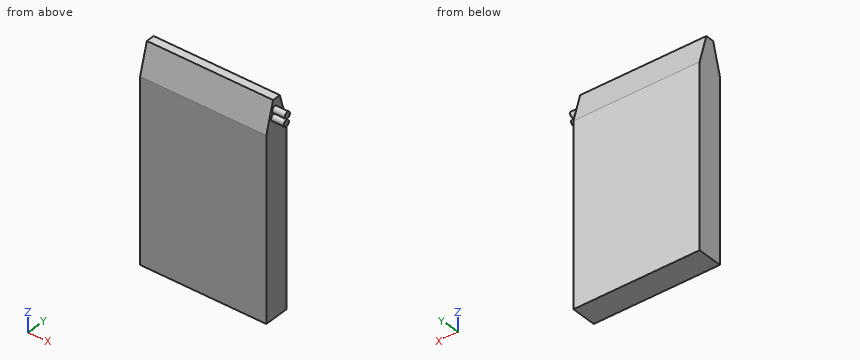
```python
from build123d import *

# Parameters (mm, degrees)
SKETCH1_W           = 30
SKETCH1_H           = 50
BOSS_EXTRUDE1_DEPTH = 6
CHAMFER1_SIZE       = 2
CHAMFER1_SIZE2      = 7
SKETCH2_R           = 0.75
BOSS_EXTRUDE2_DEPTH = 3


with BuildPart() as part:
    # Sketch1 → Boss-Extrude1 (new body)
    with BuildSketch(Plane(origin=(0, 0, 0), x_dir=(1, 0, 0), z_dir=(0, 1, 0))):
        Rectangle(SKETCH1_W, SKETCH1_H)
    extrude(amount=BOSS_EXTRUDE1_DEPTH)

    # Chamfer1
    chamfer1_edges = [part.edges().sort_by_distance(p)[0] for p in [
        (0, 0, 25),
        (0, 6, 25),
    ]]
    chamfer1_side = [part.faces().sort_by_distance(p)[0] for p in [
        (0, 3, 25),
    ]]
    chamfer(chamfer1_edges, length=CHAMFER1_SIZE, length2=CHAMFER1_SIZE2, reference=chamfer1_side[0])

    # Sketch2 → Boss-Extrude2 (add)
    with BuildSketch(Plane(origin=(15, 0, 0), x_dir=(0, 0, -1), z_dir=(1, 0, 0))):
        with Locations((-22.591828887, 2.491974932)):
            Circle(SKETCH2_R)
        with Locations((-20.930691136, 2.177979382)):
            Circle(SKETCH2_R)
    extrude(amount=BOSS_EXTRUDE2_DEPTH)


solid = part.part
```
For this review, take the finished solid that the model builds, in its own axes (mm). Coordinates: 2 decimals unless noted, no trailing zeros. Loops run counter-clockwise (first coordinate to the right, second up) from the corner with the lowest first, then second, coordinate; pieces in that order, holes last.
1. For line 1 (X direction, y = 4.5, z = 8); line 2 (Y direction, x = -6, z = 21.5), list the stretches that pass through material, from the lowest coordinate up.
2. Add section B-B, the plane z = 0. Give the boundary of the cut face in (x, y), then the cut area to 3 significant figures.
3. Add section C-C, the plane x = 16. Give the boundary of the cut face in (y, z), then the cut area to 3 significant figures.
4. Add section A-A, the plane x = -1. Give the boundary of the cut face in (y, z).
5. Add section D-D, the plane y = 4.75. Give the boundary of the cut face in (x, z) (3 decimals), then the cut area to 3 significant figures.
6. Insertion check: P1, Ø3, axis at y = 4.5, z = -5.5, coming from the +X side. The pin has a flat end and moves straight along its axis. Give the tip position at first contact, or say it passes through.
Result:
1. line 1: x = -15 to 15
1. line 2: y = 1 to 5
2. outline: (-15, 0) - (15, 0) - (15, 6) - (-15, 6) - close
2. area: 180 mm2
3. outline: circle Ø1.5 at (2.18, 20.93); circle Ø1.5 at (2.49, 22.59)
3. area: 3.53 mm2
4. outline: (0, -25) - (6, -25) - (6, 18) - (4, 25) - (2, 25) - (0, 18) - close
5. outline: (-15, -25) - (15, -25) - (15, 22.375) - (-15, 22.375) - close
5. area: 1,420 mm2
6. P1: stops at x = 15
